Geometry: final body of the model. Coordinates: model frame, mm. A direction names the side the tool comes from. Give positions to 0.01 mm unless a question says otherwise; leave off trailing zeros. Write each loop counter-clockwise with the first axis right and the second up, starting at its lowest first coordinate (ties: lowest second). Pieces come first, ordered by that corner, then holes.
Q1. Section D-D (x = 81.5). Return the cut outline in (y, z), plus the area to 3 significant figures.
Q2. Section A-A (x = -40.5). Return the cut outline in (y, z).
Q3. Pin query (flat end, axial travel): pin 1 Ø1.5 at (x, y) = (15, 1.5) entering from -Z; pin 2 Ø1 at (x, y) = (-62, 2) entering from +Z; pin 3 Ø0.9 at (x, y) = (20, 2) entering from -Z; pin 4 Ø2 at (x, z) = (-67, 25) entering from -Y. Return the tip coordinate at first contact, or that it passes through.
Q4. Line query: line 1 (Z direction, x = -71.5, y = 0.6); line 2 (Z direction, x = 86.5, y = 0.4); line 3 (Z direction, x = 8, y = 1.45). Output: solid intervals per line, ascending.
Q5. Mould query, pull axis X, two halves, no side actions, for faces 1 (the cylindrical face through (49.34, 1.48, 80.01)), 2 (the flat face through (-20, 0, -1)), 3 (the cylindrical face through (29.437, 1.479, 93.475)), 4 (the cylindrical face through (16.38, 1.48, 92.56)). Classes: +X half, -X half, draft (parallel to the pull), parting line (faces both ways), or undercut.
Q6. Section C-C (y = 0.9). State how many separate pieces and enclosed holes the cut face has, plus the area to 3 significant figures.
Q7. Section B-B (z = -38). Return the cut outline in (x, y), plus the area to 3 significant figures.
Q8. Reachability of faces 5 (the flat face through (-20, 3, -1)), 6 (the cylindrical face through (-16.38, 1.48, -92.56)) from +Z, -Z, +X, -X, +Y, -Y: full face, straight path, thin tool, end or side. Return the list, or none.
from build123d import *

# Parameters (mm, degrees)
SKETCH_1_R      = 98
EXTRUDE_1_DEPTH = 3
EXTRUDE_2_DEPTH = 3


with BuildPart() as part:
    # 草图1 → 凸台-拉伸1 (new body)
    with BuildSketch(Plane(origin=(0, 0, 0), x_dir=(1, 0, 0), z_dir=(0, 1, 0))):
        with Locations(Location((0, 0, 0), (0, 0, 270))):
            Circle(SKETCH_1_R)
        with BuildLine():
            ThreePointArc((-66.468037432, -66.468037432), (-86.457056016, -36.894138626), (-93.978720996, -2))
            Line((-93.978720996, -2), (-66.468037432, -2))
            Line((-66.468037432, -2), (-66.468037432, -66.468037432))
        make_face(mode=Mode.SUBTRACT)
        with BuildLine():
            Line((-63.468037432, -2), (-33, -2))
            Line((-33, -2), (-33, -88.017043804))
            ThreePointArc((-33, -88.017043804), (-49.129867339, -80.138980123), (-63.468037432, -69.338360412))
            Line((-63.468037432, -69.338360412), (-63.468037432, -2))
        make_face(mode=Mode.SUBTRACT)
        with BuildLine():
            Line((-30, -2), (-2, -2))
            Line((-2, -2), (-2, -93.978720996))
            ThreePointArc((-2, -93.978720996), (-16.186074601, -92.595955576), (-30, -89.084229805))
            Line((-30, -89.084229805), (-30, -2))
        make_face(mode=Mode.SUBTRACT)
        with BuildLine():
            Line((2, -93.978720996), (2, -2))
            Line((2, -2), (30, -2))
            Line((30, -2), (30, -89.084229805))
            ThreePointArc((30, -89.084229805), (16.186074601, -92.595955576), (2, -93.978720996))
        make_face(mode=Mode.SUBTRACT)
        with BuildLine():
            Line((33, -2), (63.468037432, -2))
            Line((63.468037432, -2), (63.468037432, -69.338360412))
            ThreePointArc((63.468037432, -69.338360412), (49.129867339, -80.138980123), (33, -88.017043804))
            Line((33, -88.017043804), (33, -2))
        make_face(mode=Mode.SUBTRACT)
        with BuildLine():
            ThreePointArc((93.978720996, -2), (86.457056016, -36.894138626), (66.468037432, -66.468037432))
            Line((66.468037432, -66.468037432), (66.468037432, -2))
            Line((66.468037432, -2), (93.978720996, -2))
        make_face(mode=Mode.SUBTRACT)
        with BuildLine():
            Line((-66.468037432, 2), (-93.978720996, 2))
            ThreePointArc((-93.978720996, 2), (-86.457056016, 36.894138626), (-66.468037432, 66.468037432))
            Line((-66.468037432, 66.468037432), (-66.468037432, 2))
        make_face(mode=Mode.SUBTRACT)
        with BuildLine():
            Line((-33, 2), (-63.468037432, 2))
            Line((-63.468037432, 2), (-63.468037432, 69.338360412))
            ThreePointArc((-63.468037432, 69.338360412), (-49.129867339, 80.138980123), (-33, 88.017043804))
            Line((-33, 88.017043804), (-33, 2))
        make_face(mode=Mode.SUBTRACT)
        with BuildLine():
            Line((-2, 2), (-30, 2))
            Line((-30, 2), (-30, 89.084229805))
            ThreePointArc((-30, 89.084229805), (-16.186074601, 92.595955576), (-2, 93.978720996))
            Line((-2, 93.978720996), (-2, 2))
        make_face(mode=Mode.SUBTRACT)
        with BuildLine():
            Line((30, 2), (2, 2))
            Line((2, 2), (2, 93.978720996))
            ThreePointArc((2, 93.978720996), (16.186074601, 92.595955576), (30, 89.084229805))
            Line((30, 89.084229805), (30, 2))
        make_face(mode=Mode.SUBTRACT)
        with BuildLine():
            Line((63.468037432, 2), (33, 2))
            Line((33, 2), (33, 88.017043804))
            ThreePointArc((33, 88.017043804), (49.129867339, 80.138980123), (63.468037432, 69.338360412))
            Line((63.468037432, 69.338360412), (63.468037432, 2))
        make_face(mode=Mode.SUBTRACT)
        with BuildLine():
            Line((93.978720996, 2), (66.468037432, 2))
            Line((66.468037432, 2), (66.468037432, 66.468037432))
            ThreePointArc((66.468037432, 66.468037432), (86.457056016, 36.894138626), (93.978720996, 2))
        make_face(mode=Mode.SUBTRACT)
    extrude(amount=EXTRUDE_1_DEPTH)

    # 草图2 → 凸台-拉伸2 (add)
    with BuildSketch(Plane(origin=(0, 3, 0), x_dir=(1, 0, 0), z_dir=(0, 1, 0))):
        Polygon((-66.468037432, 66.468037432), (66.468037432, 66.468037432), (63.468037432, 69.338360412), (-63.468037432, 69.338360412), align=None)
        Polygon((-66.468037432, -66.468037432), (66.468037432, -66.468037432), (63.468037432, -69.338360412), (-63.468037432, -69.338360412), align=None)
    extrude(amount=-EXTRUDE_2_DEPTH)


solid = part.part
Computed:
1. outline: (0, -54.42) - (3, -54.42) - (3, -46.84) - (0, -46.84) - close; (0, -2) - (3, -2) - (3, 2) - (0, 2) - close; (0, 46.84) - (3, 46.84) - (3, 54.42) - (0, 54.42) - close
1. area: 57.5 mm2
2. outline: (0, -89.24) - (3, -89.24) - (3, -84.83) - (0, -84.83) - close; (0, -69.34) - (3, -69.34) - (3, -66.47) - (0, -66.47) - close; (0, -2) - (3, -2) - (3, 2) - (0, 2) - close; (0, 66.47) - (3, 66.47) - (3, 69.34) - (0, 69.34) - close; (0, 84.83) - (3, 84.83) - (3, 89.24) - (0, 89.24) - close
3. pin 1: stops at z = -96.96
3. pin 2: stops at z = 76.3
3. pin 3: stops at z = -96.03
3. pin 4: stops at y = 0
4. line 1: z = -67.02 to -61.02, -2 to 2, 61.02 to 67.02
4. line 2: z = -46.06 to -36.79, -2 to 2, 36.79 to 46.06
4. line 3: z = -97.67 to -93.66, -69.34 to -66.47, -2 to 2, 66.47 to 69.34, 93.66 to 97.67
5. face 1: undercut
5. face 2: draft
5. face 3: parting line
5. face 4: undercut
6. separate pieces: 1
6. enclosed holes: 20
6. area: 6,400 mm2
7. outline: (-90.33, 0) - (-85.98, 0) - (-85.98, 3) - (-90.33, 3) - close; (-66.47, 0) - (-63.47, 0) - (-63.47, 3) - (-66.47, 3) - close; (-33, 0) - (-30, 0) - (-30, 3) - (-33, 3) - close; (-2, 0) - (2, 0) - (2, 3) - (-2, 3) - close; (30, 0) - (33, 0) - (33, 3) - (30, 3) - close; (63.47, 0) - (66.47, 0) - (66.47, 3) - (63.47, 3) - close; (85.98, 0) - (90.33, 0) - (90.33, 3) - (85.98, 3) - close
7. area: 74.1 mm2
8. face 5: +Z, -Z, +X, -X, +Y
8. face 6: +Y, -Y
